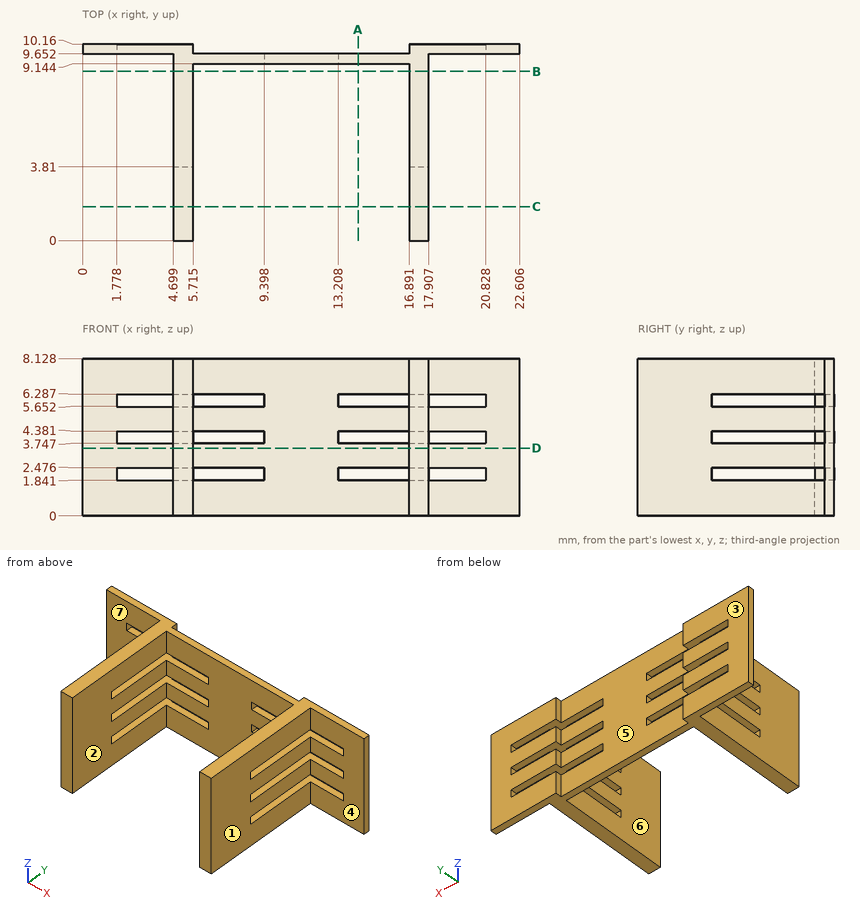
The figure shows three views and two pictorial views of one solid part (mm, origin at its lowest corner). Answer the questions. A direction names the side the tool comes from. Give positions to 0.01 mm unless a question says otherwise; leave off trailing zeros. Write each loop counter-clockwise with the first axis right and the second up, starting at its lowest first coordinate (ties: lowest second). Pieces come first, ordered by that corner, then holes. Notation, with made-up numbers: (40.5, 13.25) -> (88.5, 13.25) arc R28 ccw to (88.5, 44.25) -> close; hole circle Ø3 at (81, -34). An arc over 180 degrees is marked (long way). Use one line per item in the form item = value.
1) Straight lines are drawn through the part: probe 1 along X at (y, z) = (1.5, 5) (1 decimal); probe 2 along Z at (x, y) = (17.5, 4.25); probe 3 along Y at (x, z) = (14.75, 3.5) (1 decimal). For each, find the intervals that lie inside material, in ascending order.
Result:
probe_1 = 4.7 to 5.7, 16.9 to 17.9
probe_2 = 0 to 1.84, 2.48 to 3.75, 4.38 to 5.65, 6.29 to 8.13
probe_3 = 9.1 to 9.7
2) Section C-C on y = 1.75 is taken. Write down the section's boundary in (x, z) (1 decimal).
Result:
outline = (4.7, 0) -> (5.7, 0) -> (5.7, 8.1) -> (4.7, 8.1) -> close; (16.9, 0) -> (17.9, 0) -> (17.9, 8.1) -> (16.9, 8.1) -> close
3) Section A-A on x = 14.25 is taken. Write down the section's boundary in (y, z) (1 decimal).
Result:
outline = (9.1, 0) -> (9.7, 0) -> (9.7, 1.8) -> (9.1, 1.8) -> close; (9.1, 2.5) -> (9.7, 2.5) -> (9.7, 3.7) -> (9.1, 3.7) -> close; (9.1, 4.4) -> (9.7, 4.4) -> (9.7, 5.7) -> (9.1, 5.7) -> close; (9.1, 6.3) -> (9.7, 6.3) -> (9.7, 8.1) -> (9.1, 8.1) -> close
4) Section D-D on z = 3.5 is taken. Write down the section's boundary in (x, y) (1 decimal).
Result:
outline = (0, 9.7) -> (4.7, 9.7) -> (4.7, 0) -> (5.7, 0) -> (5.7, 9.1) -> (16.9, 9.1) -> (16.9, 0) -> (17.9, 0) -> (17.9, 9.7) -> (22.6, 9.7) -> (22.6, 10.2) -> (16.9, 10.2) -> (16.9, 9.7) -> (5.7, 9.7) -> (5.7, 10.2) -> (0, 10.2) -> close
5) A tool of negligible diameter and unlimited length cuts with its end or side. For the marked faces 4, 5, 6 and 7, from which of +Z, -Z, +X, -X, +Y, -Y can it reach the whole face along a straight path? Write none if from no direction.
Result:
face_4 = +Z, -Z, +X, -Y
face_5 = +Z, -Z, +Y
face_6 = +Z, -Z, -Y
face_7 = +Z, -Z, -X, -Y
6) Section B-B on y = 8.75 is taken. Count the separate pieces of the cut face and the enclosed holes in it.
Result:
separate_pieces = 8
enclosed_holes = 0
7) For a pull along X with two mould halves and no side action, classify the marked faces 1, 2 and 3 as +X half, -X half, draft (parallel to the pull), parting line (faces both ways), or undercut.
Result:
face_1 = +X half
face_2 = undercut
face_3 = draft
8) Each of these flat-tipped pins is pushed along its axis until it touches: P1, Ø4, axis at y = 4.5, z = 3, coming from the -X side; P2, Ø4, axis at x = 20, z = 6, coming from the -Y side; P3, Ø1, axis at x = 11.5, z = 5, coming from the -Y side. Where does it stop, or does it pass through?
Result:
P1 = 4.7
P2 = 9.65
P3 = 9.14
